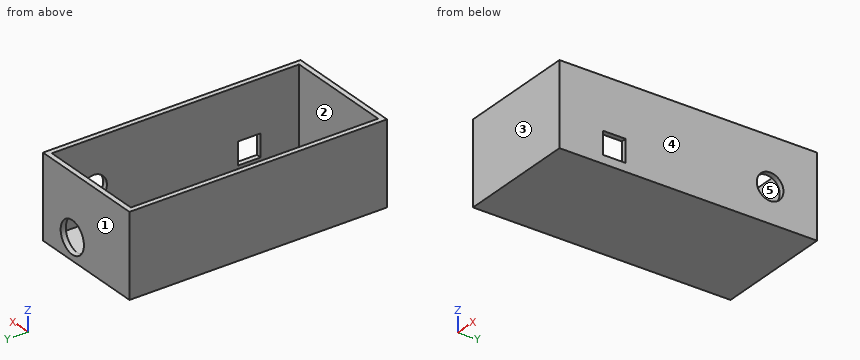
from build123d import *

# Parameters (mm, degrees)
F0_W     = 34
F0_H     = 77
F1_DEPTH = 1.6
F0_W_2   = 37.2
F0_H_2   = 80.2
F2_DEPTH = 25.6
F3_R     = 5
F4_DEPTH = 1.6
F5_R     = 4.15
F5_W     = 7
F5_H     = 7
F6_DEPTH = 1.6


with BuildPart() as f1:
    # F0 (on Top) → F1 (new body)
    with BuildSketch(Plane.XY):
        Rectangle(F0_W, F0_H)
    extrude(amount=F1_DEPTH)

    # F0 (on Top) → F2 (join)
    with BuildSketch(Plane.XY):
        Rectangle(F0_W_2, F0_H_2)
        Rectangle(F0_W, F0_H, mode=Mode.SUBTRACT)
    extrude(amount=F2_DEPTH)

    # F3 (on face) → F4 (cut, through all)
    with BuildSketch(Plane(origin=(0, 40.1, 0), x_dir=(-1, 0, 0), z_dir=(0, 1, 0))):
        with Locations((-6, 6.8)):
            Circle(F3_R)
    extrude(amount=-F4_DEPTH, mode=Mode.SUBTRACT)

    # F5 (on face) → F6 (cut, through all)
    with BuildSketch(Plane.YZ.offset(18.6)):
        with Locations((25.5, 10.8)):
            Circle(F5_R)
        with Locations((-23, 6.1)):
            Rectangle(F5_W, F5_H)
    extrude(amount=-F6_DEPTH, mode=Mode.SUBTRACT)


solid = f1.part
Can you work these out from the model? Positions are in its coordinate system, mm. Face numbers are marked on the shaded views. A direction names the side the tool comes from. Coordinates: 2 decimals unless noted, no trailing zeros. Write each loop counter-clockwise with the first axis right and the second up, starting at its lowest first coordinate (ties: lowest second). Pieces come first, ordered by that corner, then holes. Notation, with made-up numbers: (49, 40.5) -> (71, 40.5) arc R27 ccw to (71, 57.5) -> close; hole circle Ø10 at (-0.75, -9). An arc over 180 degrees is marked (long way). Write each question's results on one line, items separated by ' | '. Start each with the question number.
Q1. On a 3-axis mill with a long thin cutter (end or side, diameter ignored), from which of +Z, -Z, +X, -X, +Y, -Y can I reach the whole of each face in a straight line? I mean the marked faces 1 and 2. Say none if no direction works.
Q2. Imagine slicing it at C-C (x = 6). Write out the boundary of the cut face in (y, z), then the cut area to 3 significant figures.
Q3. If I drill on probe 1 along Y at (x, z) = (-5, 7.75); probe 2 along X at (y, z) = (4, 17.75); probe 3 along Z at (x, y) = (6, 39.55), over which ranges is the centre line in solid material (lowest first)?
Q4. I'm going to push a flat-ended pin straight in: pin 1 (4 mm diameter, centred on x = -12.5, y = -2, fed in from +Z). Where does the tip first touch, or does it pass through?
Q5. Imagine slicing it at D-D (z = 10.8). Write out the boundary of the cut face in (x, y), then the cut area to 3 significant figures.
Q6. Imagine slicing it at A-A (z = 19.75). Write out the boundary of the cut face in (x, y), then the cut area to 3 significant figures.
Q7. We'd pull the mould along Y, two halves only. Please class the marked faces 3, 4 and 5: +Y half, -Y half, draft (parallel to the pull), parting line (faces both ways), or undercut.
Q8. Imagine slicing it at B-B (y = 25.5). Write out the boundary of the cut face in (x, z), then the cut area to 3 significant figures.
Taken from the geometry:
1) face 1: +Z, -Z, +X, -X, +Y | face 2: +Z
2) outline: (-40.1, 0) -> (40.1, 0) -> (40.1, 1.8) -> (38.5, 1.8) -> (38.5, 1.6) -> (-38.5, 1.6) -> (-38.5, 25.6) -> (-40.1, 25.6) -> close; (38.5, 11.8) -> (40.1, 11.8) -> (40.1, 25.6) -> (38.5, 25.6) -> close | area: 189 mm^2
3) probe 1: y = -40.1 to -38.5, 38.5 to 40.1 | probe 2: x = -18.6 to -17, 17 to 18.6 | probe 3: z = 0 to 1.8, 11.8 to 25.6
4) pin 1: stops at z = 1.6
5) outline: (-18.6, -40.1) -> (18.6, -40.1) -> (18.6, 21.35) -> (17, 21.35) -> (17, -38.5) -> (-17, -38.5) -> (-17, 38.5) -> (3, 38.5) -> (3, 40.1) -> (-18.6, 40.1) -> close; (9, 38.5) -> (17, 38.5) -> (17, 29.65) -> (18.6, 29.65) -> (18.6, 40.1) -> (9, 40.1) -> close | area: 343 mm^2
6) outline: (-18.6, -40.1) -> (18.6, -40.1) -> (18.6, 40.1) -> (-18.6, 40.1) -> close; hole (-17, -38.5) -> (17, -38.5) -> (17, 38.5) -> (-17, 38.5) -> close | area: 365 mm^2
7) face 3: -Y half | face 4: draft | face 5: undercut
8) outline: (-18.6, 0) -> (18.6, 0) -> (18.6, 6.65) -> (17, 6.65) -> (17, 1.6) -> (-17, 1.6) -> (-17, 25.6) -> (-18.6, 25.6) -> close; (17, 14.95) -> (18.6, 14.95) -> (18.6, 25.6) -> (17, 25.6) -> close | area: 123 mm^2
